Could you check a few things on this model? Use its own coordinates, in mm. Face numbers are marked on the shaded views. A direction names the side the tool comes from. Coordinates: 2 decimals unless noted, no trailing zeros. Loops run counter-clockwise (first coordinate to the right, second up) from the corner with the lowest first, then second, coordinate; pieces in that order, holes last. Notation, with made-up numbers: (-10.5, 41) - (12.5, 41) arc R20 cw to (12.5, 69) - close; hole circle Ø5 at (18, 6). An arc over 180 degrees is marked (long way). Use CSV: the item, a comma, the result in double quotes.
from build123d import *

# Parameters (mm, degrees)
BOSS_EXTRUDE1_DEPTH = 50.8
SKETCH2_R           = 7.9375
CUT_EXTRUDE1_DEPTH  = 7.35


with BuildPart() as part:
    # Sketch1 → Boss-Extrude1 (new body)
    with BuildSketch(Plane.XY):
        Polygon((22.225, 0), (-22.225, 0), (-22.225, 44.45), (-38.1, 44.45), (-38.1, -6.35), (38.1, -6.35), (38.1, 44.45), (22.225, 44.45), align=None)
    extrude(amount=BOSS_EXTRUDE1_DEPTH)

    # Sketch2 → Cut-Extrude1 (cut, through all)
    with BuildSketch(Plane(origin=(0, 0, 0), x_dir=(1, 0, 0), z_dir=(0, 1, 0))):
        with Locations((0, -25.4)):
            Circle(SKETCH2_R)
    extrude(amount=-CUT_EXTRUDE1_DEPTH, mode=Mode.SUBTRACT)


solid = part.part
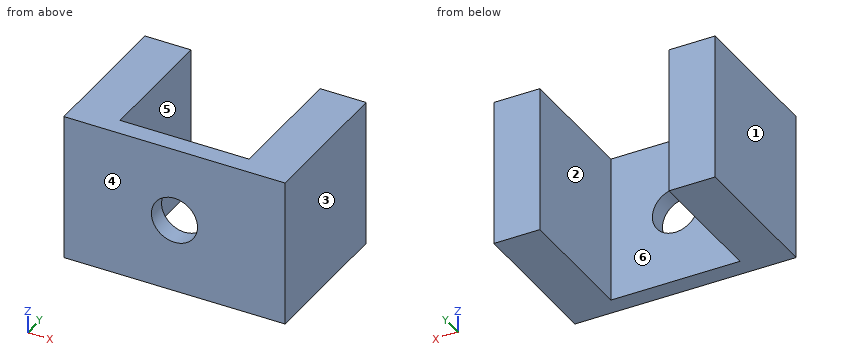
(1) Suppose I cut it at C-C (y = 39.5). Write out the boundary of the cut face in (x, z) (3 decimals).
Computed:
outline,"(-38.1, 0) - (-22.225, 0) - (-22.225, 50.8) - (-38.1, 50.8) - close; (22.225, 0) - (38.1, 0) - (38.1, 50.8) - (22.225, 50.8) - close"
(2) Suppose I cut it at D-D (y = -1.5). Write out the boundary of the cut face in (x, z) (1 decimal).
Computed:
outline,"(-38.1, 0) - (38.1, 0) - (38.1, 50.8) - (-38.1, 50.8) - close; hole circle Ø15.9 at (0, 25.4)"
(3) Please list where these lines run through material, in increasing order: line 1 (X direction, y = -5, z = 25); line 2 (X direction, y = 5.5, z = 48) (3 decimals); line 3 (Z direction, x = 0, y = -2).
Computed:
line 1,"x = -38.1 to -7.93, 7.93 to 38.1"
line 2,"x = -38.1 to -22.225, 22.225 to 38.1"
line 3,"z = 0 to 17.46, 33.34 to 50.8"
(4) Thinking about a two-plate mould opening in X: for the marked faces 3, 4, 5 and 6, which applies, +X half, -X half, draft (parallel to the pull), parting line (faces both ways), or undercut?
Computed:
face 3,"+X half"
face 4,"draft"
face 5,"undercut"
face 6,"undercut"
(5) Will these pins go through, and if not, where does the flat tip stop? pin 1 (8 mm diameter, centred on x = 12.5, z = 38.5, fed in from +Y); pin 2 (14.5 mm diameter, centred on x = 0, z = 25.4, fed in from +Y).
Computed:
pin 1,"stops at y = 0"
pin 2,"passes through"
(6) Suppose I cut it at A-A (x = 0). Write out the boundary of the cut face in (y, z).
Computed:
outline,"(-6.35, 0) - (0, 0) - (0, 17.46) - (-6.35, 17.46) - close; (-6.35, 33.34) - (0, 33.34) - (0, 50.8) - (-6.35, 50.8) - close"
(7) Which directions (+Z, -Z, +X, -X, +Y, -Y) give clear straight access to the entire face, cutting with the end or side of a thin tool? Please do the marked faces 1 and 2.
Computed:
face 1,"+Z, -Z, -X, +Y, -Y"
face 2,"+Z, -Z, +Y"
